Read the model definition and answer for the solid it produces. Units are mm, in the model's axes. A direction names the side the tool comes from. Coordinates: 2 decimals unless noted, no trailing zeros. Write each loop counter-clockwise with the first axis right and the second up, starting at its lowest first coordinate (ties: lowest second). Pieces come first, ordered by that corner, then holes. Notation, with made-up numbers: (28.5, 83.25) -> (54.5, 83.25) arc R11 cw to (54.5, 96.25) -> close; hole circle Ø10 at (73, 56.5). An arc over 180 degrees is marked (long way). Answer as a JSON object with one key per item and string values. Group by question number.
(1) Find section D-D (y = -93.75). Give the vertices of the cut face in (x, z), then the cut area to 3 significant figures.
(2) Flat-ended cylindrical pins translate along their axes: P1, Ø1.5, axis at y = -95, z = 3, coming from the -X side; P2, Ø1.6, axis at y = -92, z = -6, coming from the +X side; P3, Ø2.5, axis at x = 1.5, z = 4.5, coming from the -Y side. Find the tip coordinate at first contact, or state that the pin passes through.
(3) Which of the six approach directions +Z, -Z, +X, -X, +Y, -Y give full straight-line access (tool end or side, diameter ignored) to faces 1 (the face through (2, -96, 5.969)), 2 (the face through (-1.026, -92, -5)), 3 (the face through (-1.026, -92, 5))?
(4) For a pull along Y with two mould halves and no side action, classify faces 4 (the face through (2.33, -91.55, -6.22)), 5 (the face through (-2, -94.851, 5)), 6 (the face through (1, -96, -7.747)) as +Y half, -Y half, draft (parallel to the pull), parting line (faces both ways), or undercut.
(5) Find section C-C (y = -90.75). Count the separate pieces of the cut face and the enclosed holes in it, then the cut area to 3 significant figures.
(6) Find section A-A (z = -6.25). Give the vertices of the cut face in (x, y).
(7) Straight lines are drawn through the part: L1, parallel to X at y = -96.5, z = 4.5; L2, parallel to X at y = -95, z = 5.25; L3, parallel to Y at x = 1, z = -5.25. For each, find the intervals that lie inside material, in ascending order.
(8) Find section B-B (x = -0.75). Give the vertices of the cut face in (y, z), then the cut area to 3 significant figures.
from build123d import *

# Parameters (mm, degrees)
SKETCH1_R           = 2.794
BOSS_EXTRUDE1_DEPTH = 7.747
CUT_EXTRUDE1_START  = -5.08
SKETCH2_W           = 1.27
SKETCH2_H           = 1.27
CUT_EXTRUDE1_DEPTH  = 5.08
BOSS_EXTRUDE2_START = -1.778
BOSS_EXTRUDE2_DEPTH = 1.778
FILLET1_R           = 1.27


with BuildPart() as part:
    # Sketch1 → Boss-Extrude1 (new body)
    with BuildSketch(Plane.XY):
        with Locations(Location((-0.391227277, -94.215792273, 0), (0, 0, 180))):
            Circle(SKETCH1_R)
    extrude(amount=BOSS_EXTRUDE1_DEPTH)

    # Sketch2 → Cut-Extrude1 (cut)
    with BuildSketch(Plane.XY.offset(7.747).offset(CUT_EXTRUDE1_START)):
        with BuildLine():
            ThreePointArc((2.402772723, -94.215792273), (2.384433594, -93.896194512), (2.329656954, -93.580792273))
            Line((2.329656954, -93.580792273), (0.243772723, -93.580792273))
            Line((0.243772723, -93.580792273), (0.243772723, -94.850792273))
            Line((0.243772723, -94.850792273), (2.329656954, -94.850792273))
            ThreePointArc((2.329656954, -94.850792273), (2.384433594, -94.535390034), (2.402772723, -94.215792273))
        make_face()
        with BuildLine():
            Line((-1.026227277, -94.850792273), (-1.026227277, -93.580792273))
            Line((-1.026227277, -93.580792273), (-3.112111508, -93.580792273))
            ThreePointArc((-3.112111508, -93.580792273), (-3.166888148, -93.896194512), (-3.185227277, -94.215792273))
            ThreePointArc((-3.185227277, -94.215792273), (-3.166888148, -94.535390034), (-3.112111508, -94.850792273))
            Line((-3.112111508, -94.850792273), (-1.026227277, -94.850792273))
        make_face()
        with BuildLine():
            Line((-1.026227277, -93.580792273), (0.243772723, -93.580792273))
            Line((0.243772723, -93.580792273), (0.243772723, -91.494908041))
            ThreePointArc((0.243772723, -91.494908041), (-0.071629516, -91.440131402), (-0.391227277, -91.421792273))
            ThreePointArc((-0.391227277, -91.421792273), (-0.710825038, -91.440131402), (-1.026227277, -91.494908041))
            Line((-1.026227277, -91.494908041), (-1.026227277, -93.580792273))
        make_face()
        with BuildLine():
            Line((0.243772723, -96.936676504), (0.243772723, -94.850792273))
            Line((0.243772723, -94.850792273), (-1.026227277, -94.850792273))
            Line((-1.026227277, -94.850792273), (-1.026227277, -96.936676504))
            ThreePointArc((-1.026227277, -96.936676504), (-0.71082509, -96.991453138), (-0.391227382, -97.009792273))
            ThreePointArc((-0.391227382, -97.009792273), (-0.071629568, -96.99145315), (0.243772723, -96.936676504))
        make_face()
        with Locations((-0.391227277, -94.215792273)):
            Rectangle(SKETCH2_W, SKETCH2_H)
    extrude(amount=CUT_EXTRUDE1_DEPTH, mode=Mode.SUBTRACT)

    # Sketch3 → Boss-Extrude2 (add)
    with BuildSketch(Plane.XY.offset(7.747).offset(BOSS_EXTRUDE2_START)):
        with BuildLine():
            Line((0.243772723, -96.936676504), (0.243772723, -97.972502935))
            ThreePointArc((0.243772723, -97.972502935), (2.302849559, -96.909869109), (3.365483385, -94.850792273))
            Line((3.365483385, -94.850792273), (2.329656954, -94.850792273))
            ThreePointArc((2.329656954, -94.850792273), (1.58442907, -96.191448619), (0.243772723, -96.936676504))
        make_face()
        with BuildLine():
            Line((-1.026227277, -97.972502935), (-1.026227277, -96.936676504))
            ThreePointArc((-1.026227277, -96.936676504), (-2.366883624, -96.191448619), (-3.112111508, -94.850792273))
            Line((-3.112111508, -94.850792273), (-4.147937939, -94.850792273))
            ThreePointArc((-4.147937939, -94.850792273), (-3.085304113, -96.909869109), (-1.026227277, -97.972502935))
        make_face()
        with BuildLine():
            Line((-4.147937939, -93.580792273), (-3.112111508, -93.580792273))
            ThreePointArc((-3.112111508, -93.580792273), (-2.366883624, -92.240135926), (-1.026227277, -91.494908041))
            Line((-1.026227277, -91.494908041), (-1.026227277, -90.45908161))
            ThreePointArc((-1.026227277, -90.45908161), (-3.085304113, -91.521715436), (-4.147937939, -93.580792273))
        make_face()
        with BuildLine():
            Line((0.243772723, -90.45908161), (0.243772723, -91.494908041))
            ThreePointArc((0.243772723, -91.494908041), (1.58442907, -92.240135926), (2.329656954, -93.580792273))
            Line((2.329656954, -93.580792273), (3.365483385, -93.580792273))
            ThreePointArc((3.365483385, -93.580792273), (2.302849559, -91.521715436), (0.243772723, -90.45908161))
        make_face()
    extrude(amount=BOSS_EXTRUDE2_DEPTH)

    # Fillet1
    fillet1_edges = [part.edges().sort_by_distance(p)[0] for p in [
        (2.302849559, -96.909869109, 7.747),
        (-3.085304113, -96.909869109, 7.747),
        (-3.085304113, -91.521715436, 7.747),
        (2.302849559, -91.521715436, 7.747),
    ]]
    fillet(fillet1_edges, radius=FILLET1_R)

    # Mirror2: part across plane


with BuildPart() as part_1:
    add(part.part)
    add(part.part.mirror(Plane(origin=(-0.391227277, -94.215792273, 0), x_dir=(1, 0, 0), z_dir=(0, 0, 1))))


solid = part_1.part
Results below:
{
 "1": {"outline": "(-3.15, -2.67) -> (2.36, -2.67) -> (2.36, 2.67) -> (-3.15, 2.67) -> close", "area": "29.4 mm2"},
 "2": {"P1": "stops at x = -3.18", "P2": "stops at x = 3.15", "P3": "stops at y = -96.94"},
 "3": {"face 1": "+X, -Y", "face 2": "-Z, +Y, -Y", "face 3": "+Z, +Y, -Y"},
 "4": {"face 4": "+Y half", "face 5": "undercut", "face 6": "draft"},
 "5": {"separate pieces": "4", "enclosed holes": "0", "area": "4.15 mm2"},
 "6": {"outline": "(-4.15, -94.85) arc R3.81 ccw to (-1.03, -97.97) -> (-1.03, -94.85) -> close; (-4.15, -93.58) -> (-1.03, -93.58) -> (-1.03, -90.46) arc R3.81 ccw to start; (0.24, -97.97) arc R3.81 ccw to (3.37, -94.85) -> (0.24, -94.85) -> close; (0.24, -93.58) -> (3.37, -93.58) arc R3.81 ccw to (0.24, -90.46) -> close"},
 "7": {"L1": "x = -2 to -1.03, 0.24 to 1.22", "L2": "x = -3.07 to -1.03, 0.24 to 2.29", "L3": "y = -96.64 to -94.85, -93.58 to -91.79"},
 "8": {"outline": "(-96.99, -2.67) -> (-91.44, -2.67) -> (-91.44, 2.67) -> (-96.99, 2.67) -> close", "area": "29.6 mm2"}
}
